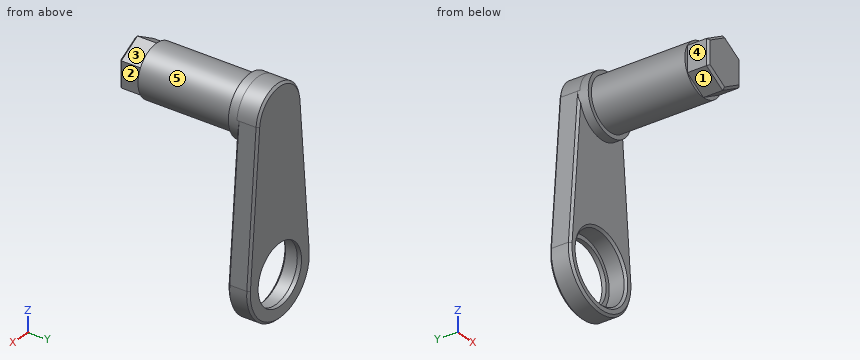
```python
from build123d import *

# Parameters (mm, degrees)
BOSS_EXTRUDE3_DEPTH = 5
BOSS_EXTRUDE1_START = 5
SKETCH2_R           = 8
BOSS_EXTRUDE1_DEPTH = 5
SKETCH3_R           = 8
SKETCH3_R_2         = 7
BOSS_EXTRUDE2_DEPTH = 1
CHAMFER1_SIZE       = 0.5


with BuildPart() as part:
    # Sketch1 → Revolve1 (revolve)
    with BuildSketch(Plane.XY, mode=Mode.PRIVATE) as revolve1_sk:
        Polygon((0, 0), (6, 0), (6, 22), (7, 22), (7, 24), (0, 24), align=None)
    revolve(revolve1_sk.sketch.rotate(Axis((0, 24, 0), (0, -1, 0)), 180), axis=Axis((0, 24, 0), (0, -1, 0)))

    # Sketch4 → Boss-Extrude3 (add)
    with BuildSketch(Plane.XZ):
        Polygon((0, 6), (-5.196152423, 3), (-5.196152423, -3), (0, -6), (5.196152423, -3), (5.196152423, 3), align=None)
    extrude(amount=BOSS_EXTRUDE3_DEPTH)

    # Sketch2 → Boss-Extrude1 (add)
    with BuildSketch(Plane(origin=(0, 24, 0), x_dir=(1, 0, 0), z_dir=(0, 1, 0)).offset(BOSS_EXTRUDE1_START)):
        with BuildLine():
            Line((-6.97423831, -0.6), (-9.963197585, 34.142857143))
            ThreePointArc((-9.963197585, 34.142857143), (0, 45), (9.963197585, 34.142857143))
            Line((9.963197585, 34.142857143), (6.97423831, -0.6))
            ThreePointArc((6.97423831, -0.6), (0, -7), (-6.97423831, -0.6))
        make_face()
        with Locations(Location((0, 35, 0), (0, 0, 180))):
            Circle(SKETCH2_R, mode=Mode.SUBTRACT)
    extrude(amount=-BOSS_EXTRUDE1_DEPTH)

    # Sketch3 → Boss-Extrude2 (add)
    with BuildSketch(Plane(origin=(0, 29, 0), x_dir=(1, 0, 0), z_dir=(0, 1, 0))):
        with Locations(Location((0, 35, 0), (0, 0, 180))):
            Circle(SKETCH3_R)
        with Locations(Location((0, 35, 0), (0, 0, 180))):
            Circle(SKETCH3_R_2, mode=Mode.SUBTRACT)
    extrude(amount=-BOSS_EXTRUDE2_DEPTH)

    # Chamfer1
    # the kernel refuses this chamfer: 0.5 mm, written as the material it takes off along each edge
    with BuildSketch(Plane(origin=(6.309723822, -5, 2.357079253), x_dir=(-0.49981095845564877, -0.027495876610585633, -0.86569797422488), z_dir=(-0.8660254037844385, 0, 0.5000000000000004)), Plane(origin=(-1.113571399, -5, -6.642920747), x_dir=(-0.4998109584556486, -0.0274958766105856, 0.8656979742248803), z_dir=(0.8660254037844386, 0, 0.5000000000000002)), Plane(origin=(5.196152423, -5, -4.285841494), x_dir=(-0.9996219169112968, -0.027495876610585647, 0), z_dir=(0, 0, 1))) as chamfer1_piece_1:
        Polygon((CHAMFER1_SIZE * 0.999621916911, -CHAMFER1_SIZE * 0.0274958766106), (-CHAMFER1_SIZE * 0.0274958766106, -CHAMFER1_SIZE * 0.999621916911), (0, 0), align=None)
    extrude(amount=8.571682988, mode=Mode.SUBTRACT)
    with BuildSketch(Plane(origin=(1.113571399, -5, 6.642920747), x_dir=(-0.013747938305293307, 0.9996219169112968, 0.02381212764409039), z_dir=(-0.8660254037844385, 0, -0.5000000000000004)), Plane(origin=(-5.196152423, -5, 4.285841494), x_dir=(-0.027495876610585647, 0.9996219169112968, 0), z_dir=(0, 0, -1)), Plane(origin=(-6.309723822, -5, -2.357079253), x_dir=(-0.013747938305292924, 0.9996219169112968, -0.023812127644089753), z_dir=(0.8660254037844386, 0, -0.5000000000000001))) as chamfer1_piece_2:
        Polygon((CHAMFER1_SIZE * 0.999621916911, CHAMFER1_SIZE * 0.0274958766106), (-CHAMFER1_SIZE * 0.0274958766106, CHAMFER1_SIZE * 0.999621916911), (0, 0), align=None)
    extrude(amount=8.571682988, mode=Mode.SUBTRACT)
    with BuildSketch(Plane(origin=(0, 24, -35), x_dir=(-1, 0, 0), z_dir=(0, 0, -1))) as chamfer1_piece_3:
        Polygon((8 + CHAMFER1_SIZE, 0), (8, CHAMFER1_SIZE), (8, 0), align=None)
    revolve(axis=Axis((0, 24, -35), (0, 1, 0)), mode=Mode.SUBTRACT)
    with BuildSketch(Plane(origin=(0, 29, 0), x_dir=(0.9963197585235825, 0, 0.08571428571428559), z_dir=(0.08571428571428559, 0, -0.9963197585235825))) as chamfer1_piece_4:
        Polygon((7, CHAMFER1_SIZE), (7 - CHAMFER1_SIZE, 0), (7, 0), align=None)
    revolve(axis=Axis((0, 29, 0), (0, -1, 0)), revolution_arc=170.165799329, mode=Mode.SUBTRACT)
    with BuildSketch(Plane(origin=(9.963197585, 29, -34.142857143), x_dir=(0.027394685145053735, -0.9996219169112968, 0.002356789423764555), z_dir=(-0.08571428571428572, 0, 0.9963197585235826)), Plane(origin=(-6.97423831, 29, 0.6), x_dir=(-0.027394685145053995, -0.9996219169112968, 0.0023567894237645753), z_dir=(-0.08571428571428566, 0, -0.9963197585235826))) as chamfer1_piece_5:
        Polygon((CHAMFER1_SIZE * 0.999621916911, -CHAMFER1_SIZE * 0.0274958766106), (-CHAMFER1_SIZE * 0.0274958766106, -CHAMFER1_SIZE * 0.999621916911), (0, 0), align=None)
    extrude(amount=34.871191548, mode=Mode.SUBTRACT)
    with BuildSketch(Plane(origin=(0, 29, -35), x_dir=(-0.9963197585235826, 0, 0.08571428571428541), z_dir=(0.08571428571428541, 0, 0.9963197585235826))) as chamfer1_piece_6:
        Polygon((10, CHAMFER1_SIZE), (10 - CHAMFER1_SIZE, 0), (10, 0), align=None)
    revolve(axis=Axis((0, 29, -35), (0, -1, 0)), revolution_arc=189.834200671, mode=Mode.SUBTRACT)
    with BuildSketch(Plane(origin=(9.963197585, 24, -34.142857143), x_dir=(-0.9959430668719438, -0.027495876610589047, -0.08568187859239684), z_dir=(-0.08571428571428572, 0, 0.9963197585235826))) as chamfer1_piece_7_section:
        Polygon((CHAMFER1_SIZE * 0.999621916911, -CHAMFER1_SIZE * 0.0274958766106), (-CHAMFER1_SIZE * 0.0274958766106, -CHAMFER1_SIZE * 0.999621916911), (0, 0), align=None)
    chamfer1_piece_7 = extrude(amount=36.157033042, mode=Mode.PRIVATE)
    chamfer1_piece_7 = chamfer1_piece_7 - Plane(origin=(0, 24.16673509, 0), x_dir=(-1, 0, 0), z_dir=(0, 1, 0)) * Cylinder(7, 75, mode=Mode.PRIVATE)
    add(chamfer1_piece_7, mode=Mode.SUBTRACT)
    with BuildSketch(Plane(origin=(0, 24, -35), x_dir=(-0.9963197585235826, 0, 0.08571428571428541), z_dir=(0.08571428571428541, 0, 0.9963197585235826))) as chamfer1_piece_8:
        Polygon((10 - CHAMFER1_SIZE, 0), (10, -CHAMFER1_SIZE), (10, 0), align=None)
    revolve(axis=Axis((0, 24, -35), (0, -1, 0)), revolution_arc=189.834200671, mode=Mode.SUBTRACT)
    with BuildSketch(Plane(origin=(-6.864023324, 24, 1.881109287), x_dir=(0.9959430668719438, -0.02749587661058904, -0.0856818785923968), z_dir=(-0.08571428571428566, 0, -0.9963197585235826))) as chamfer1_piece_9_section:
        Polygon((CHAMFER1_SIZE * 0.999621916911, -CHAMFER1_SIZE * 0.0274958766106), (-CHAMFER1_SIZE * 0.0274958766106, -CHAMFER1_SIZE * 0.999621916911), (0, 0), align=None)
    chamfer1_piece_9 = extrude(amount=36.157033042, mode=Mode.PRIVATE)
    chamfer1_piece_9 = chamfer1_piece_9 - Plane(origin=(0, 24.166735092, 0), x_dir=(-1, 0, 0), z_dir=(0, 1, 0)) * Cylinder(7, 75, mode=Mode.PRIVATE)
    add(chamfer1_piece_9, mode=Mode.SUBTRACT)


solid = part.part
```
Model file for the job. Use its own axes, mm. Face numbers are marked on the shaded views. A direction names the side the tool comes from. Give positions to 0.01 mm unless a question says otherwise; leave off trailing zeros. Write each loop counter-clockwise with the first axis right and the second up, starting at its lowest first coordinate (ties: lowest second). Pieces come first, ordered by that corner, then holes. Notation, with made-up numbers: (-15.5, 24.5) - (3.5, 24.5) arc R22 ccw to (3.5, 54.5) - close; hole circle Ø8 at (69, 1). An arc over 180 degrees is marked (long way). One line per question, with ' | ' between items. Start each with the question number.
(1) Slice it at A-A on z = -35. Write the cut outline in (x, y).
(2) Slice it at D-D on y = 4.5. Write the cut outline in (x, z).
(3) Slice it at B-B on y = 25.5. Write the cut outline in (x, z).
(4) Wall check: line 1 along Z through (x, y) = (0, 28.4); line 2 along Z through (x, y) = (0, 26.4); line 3 along Y through (x, z) = (2.25, -13). Give the ranges that are in metal, low to high. Write a range as from..to.
(5) Slice it at C-C on z = -24.5. Write the cut outline in (x, y), plus the area to 3 significant figures.
(6) Pin check, flat tips, straight feed: P1, Ø1.4, axis at y = -2.5, z = 1, coming from the +X side; P2, Ø2.5, axis at y = -2.5, z = 1, coming from the -X side; P3, Ø3, axis at x = 4, y = 19, coming from the -Z side. Stop position of each tip, or through.
(7) 3-axis set-ups, long thin cutter, end or side, ignore diameter. For the marked faces 1, 2, 3, 4 and 5: which of +Z, -Z, +X, -X, +Y, -Y reach the whole face in a straight line?
Results below:
1) outline: (-10, 24.5) - (-9.5, 24) - (-8.5, 24) - (-8, 24.5) - (-8, 28) - (-7, 28) - (-7, 29) - (-9.5, 29) - (-10, 28.5) - close; (7, 28) - (8, 28) - (8, 24.5) - (8.5, 24) - (9.5, 24) - (10, 24.5) - (10, 28.5) - (9.5, 29) - (7, 29) - close
2) outline: circle Ø12 at (0, 0)
3) outline: (-9.96, -34.14) arc R10 ccw (long way) to (9.96, -34.14) - (6.97, 0.6) arc R7 ccw to (-6.97, 0.6) - close; hole circle Ø16 at (0, -35)
4) line 1: -45..-42, -28..7 | line 2: -45..-43, -27..7 | line 3: 24..29
5) outline: (-9.13, 24.5) - (-8.63, 24) - (8.63, 24) - (9.13, 24.5) - (9.13, 28.5) - (8.63, 29) - (-8.63, 29) - (-9.13, 28.5) - close | area: 90.8 mm^2
6) P1: x = 5.2 | P2: x = -5.2 | P3: z = -5.45
7) face 1: -Z, -X, -Y | face 2: +Z, -Z, +X, -Y | face 3: +Z, +X, -Y | face 4: +Z, -Z, -X, -Y | face 5: -Y
